Answer from the drawing. Dimensions are ordinates in mm from the lowest x, y and z of the part. Give positions to 0.01 mm unless a question says otherwise; leave off trailing zeros. Order: outer loops, then holes, each group sorted by start corner. A loop starts at its lowest first (then second) coordinate and runs counter-clockwise, first axis right, second up. Notation, with made-up numbers: (-4, 77.25) -> (36, 77.25) arc R17 ccw to (36, 91.25) -> close; hole circle Ø1 at (79.25, 52.5). An arc over 180 degrees is marked (long way). One line per question, with ' | ' between items. Start each with the question number.
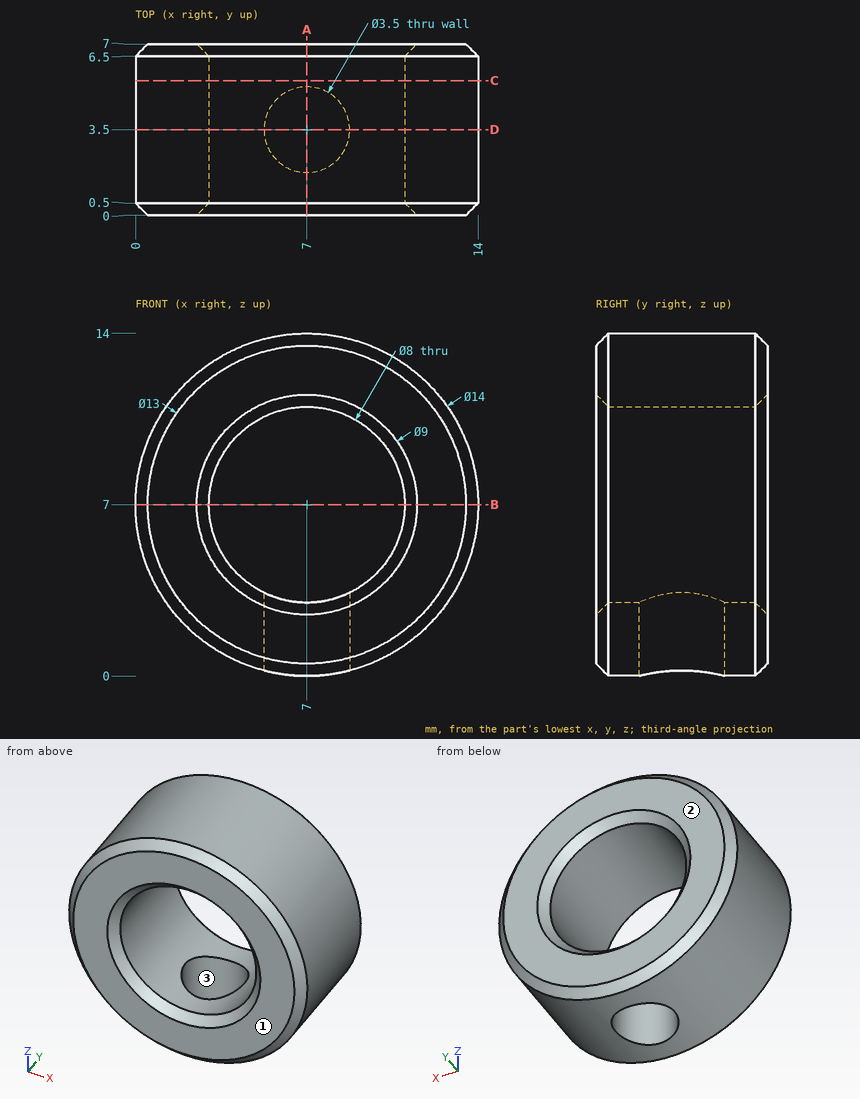
(1) The part is cut by section A-A on x = 7. Determine the outline of the cut face in (y, z).
(2) Given P1, Ø2, axis at y = 4, z = 8.5, coming from the -X side, flat-ended and moving along its own axis, determine where the tip first touches the part or whether it passes through.
(3) Determine the mould class of the marked faces 1, 2 and 3 for opening direction Y: pulls with the +Y half, pulls with the -Y half, needs draft (parallel to the pull), parting line crosses it, or undercut.
(4) The part is cut by section C-C on y = 5.5. Determine the outline of the cut face in (x, z), plus the area to 3 significant figures.
(5) The part is cut by section B-B on z = 7. Determine the outline of the cut face in (x, y).
(6) Consider line 1 (X direction, y = 2.25, z = 7); line 2 (Z direction, x = 10.25, y = 5.75); line 3 (Z direction, x = 10.5, y = 6). Determine where each line is inside the solid, lowest interval first.
(7) The part is cut by section D-D on y = 3.5. Determine the outline of the cut face in (x, z).
Result sheet:
1) outline: (0, 0.5) -> (0.5, 0) -> (1.75, 0) -> (1.75, 3) -> (0.5, 3) -> (0, 2.5) -> close; (0, 11.5) -> (0.5, 11) -> (6.5, 11) -> (7, 11.5) -> (7, 13.5) -> (6.5, 14) -> (0.5, 14) -> (0, 13.5) -> close; (5.25, 0) -> (6.5, 0) -> (7, 0.5) -> (7, 2.5) -> (6.5, 3) -> (5.25, 3) -> close
2) P1: stops at x = 0.02
3) face 1: pulls with the -Y half | face 2: pulls with the +Y half | face 3: undercut
4) outline: circle Ø14 at (7, 7); hole circle Ø8 at (7, 7) | area: 104 mm^2
5) outline: (0, 0.5) -> (0.5, 0) -> (2.5, 0) -> (3, 0.5) -> (3, 6.5) -> (2.5, 7) -> (0.5, 7) -> (0, 6.5) -> close; (11, 0.5) -> (11.5, 0) -> (13.5, 0) -> (14, 0.5) -> (14, 6.5) -> (13.5, 7) -> (11.5, 7) -> (11, 6.5) -> close
6) line 1: x = 0 to 3, 11 to 14 | line 2: z = 0.8 to 4.67, 9.33 to 13.2 | line 3: z = 0.94 to 5.06, 8.94 to 13.06
7) outline: (5.25, 0.22) -> (5.25, 3.4) arc R4 cw (long way) to (8.75, 3.4) -> (8.75, 0.22) arc R7 ccw (long way) to start
